Build history of the part. All positions in model axes, mm. A direction names the side the tool comes from. Give positions to 0.01 mm unless a question says otherwise; leave off trailing zeros. Write each loop counter-clockwise with the first axis right and the second up, starting at its lowest first coordinate (ties: lowest second). Pieces come first, ordered by that corner, then holes. Notation, with made-up numbers: M 27,2 L 80,2 A19 cw 80,34 Z; hole C -14.5,-35.75 d2. An arc over 180 degrees is marked long. One line per item, written item: value. Start each with the question number.
Autodesk Inventor part; units mm, degrees
ref_plane "Plano de correa" through (0, 189, 10) normal (0, 0, 1) x (1, 0, 0)
ref_plane "YZ Plane" through (0, 0, 0) normal (1, 0, 0) x (0, 1, 0)
ref_plane "XZ Plane" through (0, 0, 0) normal (0, 1, 0) x (-1, 0, 0)
sketch "Boceto principal" plane through (0, 0, 0) normal (1, 0, 0) x (0, 1, 0)
  line L0 (0, 20) -> (202.8, 20)
  line L1 (202.8, 20) -> (202.8, 16.356)
  line L2 (202.8, 16.356) -> (189, 12.137)
  line L3 (189, 12.137) -> (189, 7.863)
  line L4 (189, 7.863) -> (202.8, 3.644)
  line L5 (202.8, 3.644) -> (202.8, 0)
  line L6 (202.8, 0) -> (0, 0)
  line L7 (200, 15.5) -> (200, 4.5) construction
  line L8 (189, 10) -> (200, 10) construction
  line L9 (202.8, 16.356) -> (202.8, 3.644)
  line L10 (0, -4) -> (0, 24)
  line L11 (0, 0) -> (0, 20)
  dimension "d0" = 11
  dimension "d1" = 34
  dimension "d2" = 2.8
  dimension "d6" = 20
  dimension "d21" = 400
  dimension "d25" = 13.8
  dimension "d27" = 10
ref_plane "Plano de correa" through (0, 189, 10) normal (0, 0, 1) x (1, 0, 0)
revolve "Cuerpo" add sketch "Boceto principal" angle 360 about axis through (0, 0, -10) along (0, 0, 1)
revolve "Para ranuras" cut sketch "Boceto principal" angle 360 about axis through (0, 0, -10) along (0, 0, 1) contours L9 L4 L3 L2
fillet "Empalme externo" [suppressed]
fillet "Empalme interno" [suppressed]
pattern_of_one "Patrón para ranuras"
sketch "Boceto2" plane through (0, 0, 20) normal (0, 0, 1) x (1, 0, 0)
  point P0 (0, 0)
  point P1 (0, 0)
hole "Agujero1" at (0, 0, 20) direction (0, 0, -1) diameter 15 end through all
equation "\"d0\" = da_Bw"
equation "\"d1\" = da_Alfa"
equation "\"d2\" = da_c"
equation "\"d21\" = da_Dw"
equation "\"d25\" = da_Hd"
equation "\"d27\" = da_Se"
equation "\"da_r1\" = 0"
equation "\"da_r2\" = 0"
equation "\"d18\" = da_Sg"
equation "\"da_Bw\" = 11"
equation "\"da_Alfa\" = 34deg"
equation "\"da_c\" = 2.8"
equation "\"da_Dw\" = 400"
equation "\"da_Hd\" = 13.8"
equation "\"da_Se\" = 10"
equation "\"da_Sg\" = 15"
properties part number "Polea ranurada2" material "Steel"
1) Band-saw the part on A-A (y = 0). List the corners of the cut face in (x, z), then the cut area to 3 significant figures.
2) Probe line 1 along X through (y, z) = (0, 10.75); line 2 along Z through (x, y) = (-158, -104). List the from-to ranges inside material, lowest first. Write a range as from..to.
3) Mould opens along Y. For faces 1 (the face through (-0.33, 7.493, 9.86)), 2 (the face through (-3, 42, 0)), 3 (the face through (60.916, 193.435, 18.152)) say: released by +Y, released by -Y, zero draft, split by the parting line, or undercut.
4) Drop flat-ended pins along their axis: P1, Ø6, axis at x = -94.5, z = 4, coming from the +Y side; P2, Ø4, axis at y = -3, z = 14.5, coming from the -X side; P3, Ø5, axis at y = -35.5, z = 16, coming from the -X side. Give the stop position or say it passes through.
5) Tool access for faces 4 (the face through (-3, 42, 20)), 5 (the face through (-185.35, -41.16, 7.6)): list every direction of +Z, -Z, +X, -X, +Y, -Y with a clear straight run to the whole face (end or side of a thin tool).
Model answer:
1. outline: M -202.8,0 L -7.5,0 L -7.5,20 L -202.8,20 L -202.8,16.36 L -189,12.14 L -189,7.86 L -202.8,3.64 Z; M 7.5,0 L 202.8,0 L 202.8,3.64 L 189,7.86 L 189,12.14 L 202.8,16.36 L 202.8,20 L 7.5,20 Z
1. area: 7,580 mm²
2. line 1: x = -189..-7.5, 7.5..189
2. line 2: z = 0..7.82, 12.18..20
3. face 1: undercut
3. face 2: zero draft
3. face 3: split by the parting line
4. P1: stops at y = 180.97
4. P2: stops at x = -202.79
4. P3: stops at x = -200.09
5. face 4: +Z, +X, -X, +Y, -Y
5. face 5: none
